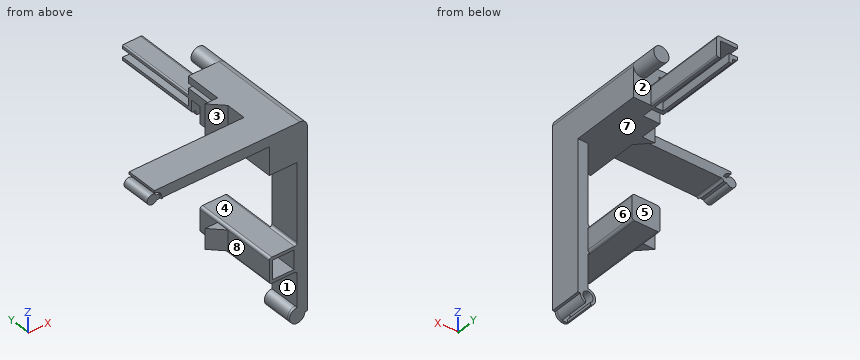
```python
from build123d import *
from build123d.topology import SkipClean

# Parameters (mm, degrees)
SKETCH1_W                 = 30
SKETCH1_H                 = 30
BOSS_EXTRUDE1_DEPTH       = 80
SKETCH2_R                 = 6
BOSS_EXTRUDE2_DEPTH       = 20
CUT_EXTRUDE1_DEPTH        = 83.764726786
BOSS_EXTRUDE3_DEPTH       = 65
BOSS_EXTRUDE5_DEPTH       = 2
BOSS_EXTRUDE6_DEPTH       = 23
BOSS_EXTRUDE7_DEPTH       = 25
FILLET1_R                 = 2
SKETCH11_R                = 6.055782361
CUT_EXTRUDE2_DEPTH        = 2.125
SKETCH12_W                = 13.25
SKETCH12_H                = 8.5
CUT_EXTRUDE3_DEPTH        = 13.25
FILLET2_R                 = 2
CUT_EXTRUDE4_REACH        = 195.534
SKETCH14_W                = 3.75
SKETCH14_H                = 3.75
FILLET3_R                 = 1
SKETCH15_W                = 10
SKETCH15_H                = 4
CUT_EXTRUDE5_DEPTH        = 25
BOSS_EXTRUDE8_REACH       = 230.211
SKETCH17_W                = 22
SKETCH17_H                = 20
SKETCH18_W                = 17
SKETCH18_H                = 15
CUT_EXTRUDE6_DEPTH        = 66
FILLET4_R                 = 2
FILLET5_R                 = 2
CHAMFER1_SIZE             = 7
BOSS_EXTRUDE9_DEPTH       = 30
BOSS_EXTRUDE10_DEPTH      = 8
BOSS_EXTRUDE10_DEPTH_BACK = 8


with BuildPart() as part:
    # Sketch1 → Boss-Extrude1 (new body)
    with BuildSketch(Plane(origin=(0, 0, 0), x_dir=(1, 0, 0), z_dir=(0, 1, 0))):
        Rectangle(SKETCH1_W, SKETCH1_H)
    extrude(amount=BOSS_EXTRUDE1_DEPTH)

    # Sketch2 → Boss-Extrude2 (add)
    with BuildSketch(Plane(origin=(0, 80, 0), x_dir=(1, 0, 0), z_dir=(0, 1, 0))):
        with Locations(Location((9, -9, 0), (0, 0, 270))):
            Circle(SKETCH2_R)
    extrude(amount=BOSS_EXTRUDE2_DEPTH)

    # Sketch3 → Cut-Extrude1 (cut, through all)
    with BuildSketch(Plane(origin=(0, 80, 0), x_dir=(1, 0, 0), z_dir=(0, 1, 0))):
        with BuildLine():
            Line((9, -15), (15, -15))
            Line((15, -15), (15, -9))
            ThreePointArc((15, -9), (13.242640687, -13.242640687), (9, -15))
        make_face()
    extrude(amount=-CUT_EXTRUDE1_DEPTH, mode=Mode.SUBTRACT)

    # Sketch4 → Boss-Extrude3 (add)
    with BuildSketch(Plane(origin=(0, 80, 0), x_dir=(1, 0, 0), z_dir=(0, 1, 0))):
        Polygon((-8.25, 11.25), (-8.25, 8.25), (-11.25, 8.25), (-15, 8.25), (-15, 11.25), (-11.25, 11.25), (-11.25, 15), (-8.25, 15), align=None)
        Polygon((-1.75, 1.75), (-11.25, 1.75), (-15, 1.75), (-15, -1.25), (-11.25, -1.25), (1.25, -1.25), (1.25, 11.25), (1.25, 15), (-1.75, 15), (-1.75, 11.25), align=None)
    extrude(amount=BOSS_EXTRUDE3_DEPTH)

    # Sketch6 → Boss-Extrude5 (add)
    with BuildSketch(Plane.XZ):
        with BuildLine():
            Line((15, -15), (7, -15))
            Line((7, -15), (7, -126.175))
            ThreePointArc((7, -126.175), (2.757359313, -136.417640687), (13, -132.175))
            Line((13, -132.175), (15, -132.175))
            Line((15, -132.175), (15, -15))
        make_face()
    extrude(amount=-BOSS_EXTRUDE5_DEPTH)

    # Sketch7 → Boss-Extrude6 (add)
    with SkipClean():  # the faces are left unmerged after this step: merging them gives an invalid solid
        with BuildSketch(Plane(origin=(0, 2, 0), x_dir=(1, 0, 0), z_dir=(0, 1, 0))):
            with BuildLine():
                Line((9, 137.831854249), (9, 135.639101615))
                ThreePointArc((9, 135.639101615), (7, 128.175), (5, 135.639101615))
                Line((5, 135.639101615), (5, 137.831854249))
                ThreePointArc((5, 137.831854249), (1.086408642, 131.160388128), (7, 126.175))
                Line((7, 126.175), (7, 15))
                Line((7, 15), (15, 15))
                Line((15, 15), (15, 132.175))
                Line((15, 132.175), (13, 132.175))
                ThreePointArc((13, 132.175), (11.898979486, 135.639101615), (9, 137.831854249))
            make_face()
        extrude(amount=BOSS_EXTRUDE6_DEPTH)

    # Sketch9 → Boss-Extrude7 (add)
    with SkipClean():  # the faces are left unmerged after this step: merging them gives an invalid solid
        with BuildSketch(Plane.XZ):
            with BuildLine():
                Line((-15, 15), (-15, 7))
                Line((-15, 7), (-99.5, 7))
                ThreePointArc((-99.5, 7), (-99.577697751, 6.037536458), (-99.80877869, 5.1))
                Line((-99.80877869, 5.1), (-102.122778509, 5.1))
                ThreePointArc((-102.122778509, 5.1), (-109.375, 7), (-102.122778509, 8.9))
                Line((-102.122778509, 8.9), (-99.625, 8.9))
                ThreePointArc((-99.625, 8.9), (-101.816885554, 11.955834237), (-105.375001601, 13.173329766))
                Line((-105.375001601, 13.173329766), (-105.375001601, 15))
                Line((-105.375001601, 15), (-15, 15))
            make_face()
        extrude(amount=-BOSS_EXTRUDE7_DEPTH)

    # Fillet1
    fillet1_edges = [part.edges().sort_by_distance(p)[0] for p in [
        (-99.5, 12.5, 7),
    ]]
    fillet(fillet1_edges, radius=FILLET1_R)

    # Sketch11 → Cut-Extrude2 (cut)
    with SkipClean():  # the faces are left unmerged after this step: merging them gives an invalid solid
        with BuildSketch(Plane.XZ):
            with Locations((-105.5, 7)):
                Circle(SKETCH11_R)
        extrude(amount=-CUT_EXTRUDE2_DEPTH, mode=Mode.SUBTRACT)

    # Sketch12 → Cut-Extrude3 (cut)
    with SkipClean():  # the faces are left unmerged after this step: merging them gives an invalid solid
        with BuildSketch(Plane(origin=(0, 0, -15), x_dir=(-1, 0, 0), z_dir=(0, 0, -1))):
            with Locations((8.375, 72.75)):
                Rectangle(SKETCH12_W, SKETCH12_H)
        extrude(amount=-CUT_EXTRUDE3_DEPTH, mode=Mode.SUBTRACT)

    # Fillet2
    fillet2_edges = [part.edges().sort_by_distance(p)[0] for p in [
        (1.25, 112.5, 1.25),
    ]]
    fillet(fillet2_edges, radius=FILLET2_R)

    # Sketch14 → Cut-Extrude4 (cut, up to next)
    with BuildSketch(Plane(origin=(0, 80, 0), x_dir=(1, 0, 0), z_dir=(0, 1, 0)), mode=Mode.PRIVATE) as cut_extrude4_sk1:
        with Locations((-13.125, 13.125)):
            Rectangle(SKETCH14_W, SKETCH14_H)
    cut_extrude4_tool1 = extrude(cut_extrude4_sk1.sketch, amount=-CUT_EXTRUDE4_REACH, mode=Mode.PRIVATE) & part.part
    add(cut_extrude4_tool1.solids().sort_by_distance((-13.125, 80, -13.125))[0], mode=Mode.SUBTRACT)

    # Fillet3
    fillet3_edges = [part.edges().sort_by_distance(p)[0] for p in [
        (-11.25, 112.5, -15),
        (-11.25, 112.5, -11.25),
        (-15, 112.5, -11.25),
        (-15, 112.5, 1.25),
        (1.25, 112.5, -15),
    ]]
    fillet(fillet3_edges, radius=FILLET3_R)

    # Sketch15 → Cut-Extrude5 (cut)
    with SkipClean():  # the faces are left unmerged after this step: merging them gives an invalid solid
        with BuildSketch(Plane(origin=(0, 80, 0), x_dir=(1, 0, 0), z_dir=(0, 1, 0))):
            with Locations((-10, -7.625)):
                Rectangle(SKETCH15_W, SKETCH15_H)
        extrude(amount=-CUT_EXTRUDE5_DEPTH, mode=Mode.SUBTRACT)

    # Boss-Extrude8: up to this face of the body (flat: up to its plane)
    boss_extrude8_end = Plane(part.part.faces().sort_by_distance((-8.375, 68.5, -8.375))[0])
    # Sketch17 → Boss-Extrude8 (add, up to the picked face)
    with BuildSketch(Plane.XZ, mode=Mode.PRIVATE) as boss_extrude8_sk1:
        with Locations((-4, -88.38125)):
            Rectangle(SKETCH17_W, SKETCH17_H)
    boss_extrude8_tool1 = split(extrude(boss_extrude8_sk1.sketch, amount=-BOSS_EXTRUDE8_REACH, mode=Mode.PRIVATE), bisect_by=boss_extrude8_end, keep=Keep.BOTH, mode=Mode.PRIVATE)
    add(boss_extrude8_tool1.solids().sort_by(Axis((-4, 0, -88.38125), (0, 1, 0)))[0])

    # Sketch18 → Cut-Extrude6 (cut)
    with SkipClean():  # the faces are left unmerged after this step: merging them gives an invalid solid
        with BuildSketch(Plane.XZ):
            with Locations((-4, -88.38125)):
                Rectangle(SKETCH18_W, SKETCH18_H)
        extrude(amount=-CUT_EXTRUDE6_DEPTH, mode=Mode.SUBTRACT)

    # Fillet4
    fillet4_edges = [part.edges().sort_by_distance(p)[0] for p in [
        (7, 13.5, -78.38125),
        (7, 13.5, -98.38125),
        (-15, 34.25, -98.38125),
        (-15, 34.25, -78.38125),
    ]]
    fillet(fillet4_edges, radius=FILLET4_R)

    # Fillet5
    fillet5_edges = [part.edges().sort_by_distance(p)[0] for p in [
        (7, 46.75, -78.38125),
        (7, 46.75, -98.38125),
    ]]
    fillet(fillet5_edges, radius=FILLET5_R)

    # Chamfer1
    chamfer1_edges = [part.edges().sort_by_distance(p)[0] for p in [
        (-12.5, 66, -88.38125),
        (-4, 66, -80.88125),
        (4.5, 66, -88.38125),
        (-4, 66, -95.88125),
    ]]
    chamfer(chamfer1_edges, length=CHAMFER1_SIZE)

    # Sketch19 → Boss-Extrude9 (add)
    with SkipClean():  # the faces are left unmerged after this step: merging them gives an invalid solid
        with BuildSketch(Plane.XY.offset(15)):
            Polygon((-15, 41), (-15, 51), (-25, 51), align=None)
        extrude(amount=-BOSS_EXTRUDE9_DEPTH)

    # Sketch20 → Boss-Extrude10 (add, two sides: drawn at the far end of the back side and taken through both)
    with SkipClean():  # the faces are left unmerged after this step: merging them gives an invalid solid
        with BuildSketch(Plane.XY.offset(-88.38125).offset(-BOSS_EXTRUDE10_DEPTH_BACK)):
            Polygon((-15, 41), (-15, 51), (-25, 51), align=None)
        extrude(amount=BOSS_EXTRUDE10_DEPTH + BOSS_EXTRUDE10_DEPTH_BACK)


solid = part.part
```
Here's how the part is built. I have some questions about the finished solid (model axes, mm). Face numbers are marked on the shaded views. A direction names the side the tool comes from. Give positions to 0.01 mm unless a question says otherwise; leave off trailing zeros. Loops run counter-clockwise (first coordinate to the right, second up) from the corner with the lowest first, then second, coordinate; pieces in that order, holes last. Notation, with made-up numbers: M 84.25,-20.5 L 135.25,-20.5 A21 ccw 135.25,1.5 Z; hole C -25,-3.75 d5. An arc over 180 degrees is marked long. Put each result on its own line as item: value. Start each with the question number.
(1) I want a section at B-B on y = 134. Please give me the cut outline in (x, z), then the cut area to 3 significant figures.
(2) For the marked faces 4, 5, 6, 7 and 8, which set-ups out of +Z, -Z, +X, -X, +Y, -Y let a thin tool reach every point of the face, with its end or its side?
(3) I need wall thicknesses on line 1 along X through (y, z) = (59, -13); line 2 along X through (y, z) = (59, -95.5); line 3 along X through (y, z) = (9, -124.5). Which ranges of each line are inside material? Lowest first, please. Write a range as [from, to].
(4) If we mould it in two halves opening along Y, with no side actions, what happens to the marked faces 1, 2 and 3? For each: +Y half, -Y half, draft (parallel to the pull), parting line (faces both ways), or undercut.
(5) I want a section at C-C on z = -85.5. Please give me the cut outline in (x, y), then the cut area to 3 significant figures.
(6) I want a section at A-A on y = 27. Please give me the cut outline in (x, z).
(7) Will these pins go through, and if not, where does the flat tip stop? pin 1 Ø24 at (y, z) = (104.5, 6.5) entering from -X; pin 2 Ø20 at (y, z) = (14, -118) entering from -X; pin 3 Ø3.5 at (x, z) = (-60.5, 9) entering from +Y; pin 4 Ø24 at (y, z) = (26.5, 2) entering from -X (3 decimals).
(8) I want a section at D-D on x = -63. Please give me the cut outline in (y, z), then the cut area to 3 significant figures.
Answer block:
1. outline: M -15,-10.25 A1 ccw -14,-11.25 L -12.25,-11.25 A1 cw -11.25,-12.25 L -11.25,-14 A1 ccw -10.25,-15 L -8.25,-15 L -8.25,-8.25 L -15,-8.25 Z; M -15,-1.75 L -1.75,-1.75 L -1.75,-15 L 0.25,-15 A1 ccw 1.25,-14 L 1.25,-0.75 A2 ccw -0.75,1.25 L -14,1.25 A1 ccw -15,0.25 Z
1. area: 118 mm^2
2. face 4: -X, +Y, -Y
2. face 5: -Z, +X, -X, +Y
2. face 6: -Z, +X, +Y
2. face 7: -X, +Y
2. face 8: -Z, -X, -Y
3. line 1: [-15, 15]
3. line 2: [-15, -12.5], [4.5, 7]
3. line 3: [7, 15]
4. face 1: draft
4. face 2: +Y half
4. face 3: undercut
5. outline: M -25,51 L -15,41 L -15,0 L -12.5,0 L -12.5,59 L -7.88,63.62 L -0.12,63.62 L 4.5,59 L 4.5,0 L 15,0 L 15,25 L 7,25 L 7,68.5 L -15,68.5 L -15,51 Z
5. area: 697 mm^2
6. outline: M -15,-96.38 A2 ccw -13,-98.38 L 5,-98.38 A2 ccw 7,-96.38 L 7,-80.38 A2 ccw 5,-78.38 L -13,-78.38 A2 ccw -15,-80.38 Z; M -15,-15 L 15,-15 L 15,9 A6 ccw 9,15 L -15,15 Z; hole M -12.5,-95.88 L 4.5,-95.88 L 4.5,-80.88 L -12.5,-80.88 Z
7. pin 1: x = -15
7. pin 2: x = 2.69
7. pin 3: y = 25
7. pin 4: x = -109.375
8. outline: M 0,7 L 25,7 L 25,15 L 0,15 Z
8. area: 200 mm^2
